The model under review builds one solid part; all positions refer to its coordinate system, in mm. Round coordinates to 2 decimals unless told otherwise and drop trailing zeros. Order: outer loops, then holes, each group sorted by start corner. A loop starts at its lowest first (then second) coordinate and runs counter-clockwise, first axis right, second up. Notation, with made-up numbers: M 78,32.5 L 91,32.5 A5 ccw 91,39.5 Z; hole C -38,55 d6. An arc over 180 degrees is marked long. Answer as a JSON object with one key per item and string values. Group by question number.
1. Add section C-C on y = 2.6. State the section outline as (x, z) points (3 decimals), and give its area (3 significant figures).
2. Add section B-B on z = 0. State the section outline as (x, y) points.
3. To check wall thickness, follow probe 1 along Z at (x, y) = (0, 4.05); probe 2 along Z at (x, y) = (-2.5, 1.5); probe 3 along X at (y, z) = (1.9, -10). State the ranges of each line that lie inside material, in increasing order. Write a range as [from, to].
4. Add section D-D on x = 37. State the section outline as (y, z) points, and give its area (3 significant figures).
5. Clearance check with flat-ended pins moving along their axes: P1, Ø19, axis at x = 0, z = 50, coming from the -Y side; P2, Ø1.5, axis at y = 2.5, z = -14, coming from the +X side; P3, Ø1, axis at y = 1.5, z = -1, coming from the -X side; P4, Ø1.5, axis at x = 12, y = 4, coming from the +Z side. State where each tip first meets the part, or that it passes through.
6. Add section A-A on x = -52. State the section outline as (y, z) points, and give its area (3 significant figures).
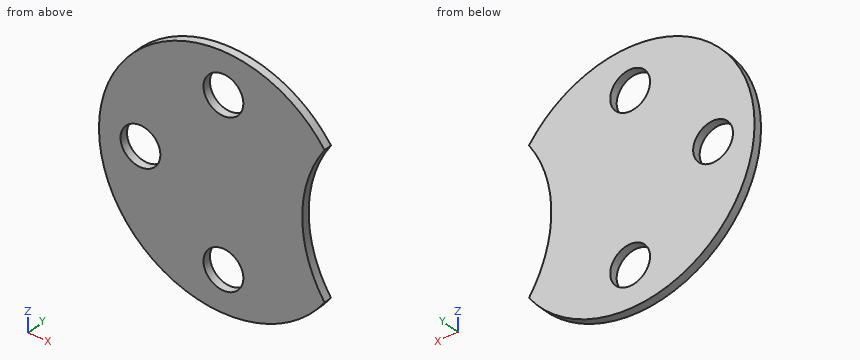
```python
from build123d import *

# Parameters (mm, degrees)
SKETCH_1_R          = 75
EXTRUDE_1_DEPTH     = 5
HOLE_WIZARD_1_D     = 24
SKETCH_4_R          = 77.5
CUT_EXTRUDE_1_DEPTH = 5


with BuildPart() as part:
    # 草图1 → 凸台-拉伸1 (new body)
    with BuildSketch(Plane(origin=(0, 0, 0), x_dir=(1, 0, 0), z_dir=(0, 1, 0))):
        with Locations(Location((0, 0, 0), (0, 0, 270))):
            Circle(SKETCH_1_R)
    extrude(amount=EXTRUDE_1_DEPTH)

    # 孔1 (through all)
    with Locations(Plane.XZ):
        with Locations((0, 50), (0, -50), (-50, 0)):
            Hole(HOLE_WIZARD_1_D / 2)

    # 草图4 → 切除-拉伸1 (cut)
    with BuildSketch(Plane.XZ):
        with Locations((125, 0)):
            Circle(SKETCH_4_R)
    extrude(amount=-CUT_EXTRUDE_1_DEPTH, mode=Mode.SUBTRACT)


solid = part.part
```
Recorded:
{
 "1": {"outline": "M 60.975,-43.67 A77.5 cw 60.975,43.67 A75 ccw long Z; hole C -50,0 d24; hole C 0,-50 d24; hole C 0,50 d24", "area": "14,700 mm²"},
 "2": {"outline": "M -75,0 L -62,0 L -62,5 L -75,5 Z; M -38,0 L 47.5,0 L 47.5,5 L -38,5 Z"},
 "3": {"probe 1": "z = [-75, -62], [-38, 38], [62, 75]", "probe 2": "z = [-74.96, -61.74], [-38.26, 38.26], [61.74, 74.96]", "probe 3": "x = [-74.33, -56.63], [-43.37, 48.15]"},
 "4": {"outline": "M 0,-65.24 L 5,-65.24 L 5,65.24 L 0,65.24 Z", "area": "652 mm²"},
 "5": {"P1": "passes through", "P2": "stops at x = 48.92", "P3": "stops at x = -75", "P4": "stops at z = 74.15"},
 "6": {"outline": "M 0,-54.05 L 5,-54.05 L 5,-11.83 L 0,-11.83 Z; M 0,11.83 L 5,11.83 L 5,54.05 L 0,54.05 Z", "area": "422 mm²"}
}
